Work out the finished part from the listing and answer in its coordinate system (mm). A direction names the side the tool comes from. Round coordinates to 2 decimals unless told otherwise and drop trailing zeros. Loops run counter-clockwise (first coordinate to the right, second up) from the corner with the lowest first, then second, coordinate; pieces in that order, holes last.
```python
from build123d import *

# Parameters (mm, degrees)
SKETCH1_R           = 40
BOSS_EXTRUDE1_DEPTH = 200
SKETCH2_R           = 10
CUT_EXTRUDE1_DEPTH  = 120
CUT_EXTRUDE2_START  = -120
SKETCH3_R           = 10
CUT_EXTRUDE2_DEPTH  = 120


with BuildPart() as part:
    # Sketch1 → Boss-Extrude1 (new, symmetric)
    with BuildSketch(Plane.XY):
        Circle(SKETCH1_R)
    extrude(amount=BOSS_EXTRUDE1_DEPTH, both=True)

    # Sketch2 → Cut-Extrude1 (cut)
    with BuildSketch(Plane.XY.offset(200)):
        Circle(SKETCH2_R)
    extrude(amount=-CUT_EXTRUDE1_DEPTH, mode=Mode.SUBTRACT)

    # Sketch3 → Cut-Extrude2 (cut)
    with BuildSketch(Plane(origin=(0, 0, -200), x_dir=(-1, 0, 0), z_dir=(0, 0, -1)).offset(CUT_EXTRUDE2_START)):
        with Locations(Location((0, 0, 0), (0, 0, 180))):
            Circle(SKETCH3_R)
    extrude(amount=CUT_EXTRUDE2_DEPTH, mode=Mode.SUBTRACT)


solid = part.part
```
1. Given pin 1 (10 mm diameter, centred on y = -27.5, z = 118, fed in from -X); pin 2 (6 mm diameter, centred on y = 20, z = -79.5, fed in from +X); pin 3 (1 mm diameter, centred on x = -18, z = 21, fed in from -Y); pin 4 (10 mm diameter, centred on x = 3.5, y = 4, fed in from -Z), each flat-ended and moving along its own axis, determine where each tip first touches the part or whether it passes through.
Answer key:
pin 1: stops at x = -33.07
pin 2: stops at x = 36.21
pin 3: stops at y = -35.97
pin 4: stops at z = -200
2. Consider probe 1 along Y at (x, z) = (0, -159); probe 2 along Y at (x, z) = (1, -159); probe 3 along X at (y, z) = (9, 141.5). Determine where each line is inside the solid, lowest interval first.
Answer key:
probe 1: y = -40 to -10, 10 to 40
probe 2: y = -39.99 to -9.95, 9.95 to 39.99
probe 3: x = -38.97 to -4.36, 4.36 to 38.97
3. Which of the six approach directions +Z, -Z, +X, -X, +Y, -Y give full straight-line access (tool end or side, diameter ignored) to faces 4 (the face through (-2.17, -9.76, 140.84)), 5 (the face through (8, -8, -200)), 6 (the face through (-10, 0, -139))?
Answer key:
face 4: +Z
face 5: -Z, +X, -X, +Y, -Y
face 6: -Z
4. Find section A-A (z = -116). Write down the section's boundary in (x, y).
Answer key:
outline: circle Ø80 at (0, 0); hole circle Ø20 at (0, 0)
5. Determine the mould class of faces 1 (the face through (8, -8, 200)), 2 (the face through (0, 0, 80)), 3 (the face through (-8.67, -39.05, 2.8)) for opening direction Y: +Y half, -Y half, draft (parallel to the pull), parting line (faces both ways), or undercut.
Answer key:
face 1: draft
face 2: undercut
face 3: parting line
6. Find section D-D (z = 54). Write down the section's boundary in (x, y), then the cut area to 3 significant figures.
Answer key:
outline: circle Ø80 at (0, 0)
area: 5,030 mm2
7. Find section B-B (x = 0). Write down the section's boundary in (y, z).
Answer key:
outline: (-40, -200) - (-10, -200) - (-10, -80) - (10, -80) - (10, -200) - (40, -200) - (40, 200) - (10, 200) - (10, 80) - (-10, 80) - (-10, 200) - (-40, 200) - close
